from build123d import *

# Parameters (mm, degrees)
BOSS_EXTRUDE1_DEPTH = 100
SKETCH2_R           = 4
BOSS_EXTRUDE2_DEPTH = 5
CUT_EXTRUDE1_DEPTH  = 111.145358504
BOSS_EXTRUDE3_DEPTH = 20
SKETCH6_W           = 16
SKETCH6_H           = 82.013760225
CUT_EXTRUDE2_DEPTH  = 20
FILLET1_R           = 2
SKETCH7_W           = 20
SKETCH7_H           = 90.042878707
SKETCH7_W_2         = 16
SKETCH7_H_2         = 66.692206804
BOSS_EXTRUDE4_DEPTH = 15
CHAMFER1_SIZE       = 8


with BuildPart() as part:
    # Sketch1 → Boss-Extrude1 (new body)
    with BuildSketch(Plane.XY):
        Polygon((28, 4), (44, 4), (44, 9), (-16, 9), (-16, 4), (0, 4), (0, 0), (28, 0), align=None)
    extrude(amount=BOSS_EXTRUDE1_DEPTH)

    # Sketch2 → Boss-Extrude2 (add)
    with BuildSketch(Plane.XY.offset(100)):
        with BuildLine():
            Line((6, 15), (6, 0))
            Line((6, 0), (22, 0))
            Line((22, 0), (22, 15))
            ThreePointArc((22, 15), (14, 23), (6, 15))
        make_face()
        with Locations((14, 15)):
            Circle(SKETCH2_R, mode=Mode.SUBTRACT)
    extrude(amount=-BOSS_EXTRUDE2_DEPTH)

    # Sketch3 → Cut-Extrude1 (cut, through all)
    with BuildSketch(Plane(origin=(0, 9, 0), x_dir=(1, 0, 0), z_dir=(0, 1, 0))):
        Polygon((36, -100), (44, -88), (44, -100), align=None)
        Polygon((-8, -100), (-16, -100), (-16, -88), align=None)
    extrude(amount=-CUT_EXTRUDE1_DEPTH, mode=Mode.SUBTRACT)

    # Sketch5 → Boss-Extrude3 (add)
    with BuildSketch(Plane(origin=(0, 9, 0), x_dir=(1, 0, 0), z_dir=(0, 1, 0))):
        Polygon((-16, 0), (0, 0), (0, -5.756429966), (28.329099736, -5.756429966), (28.329099736, 0), (44, 0), (44, -12.986239775), (-16, -12.986239775), align=None)
    extrude(amount=BOSS_EXTRUDE3_DEPTH)

    # Sketch6 → Cut-Extrude2 (cut)
    with BuildSketch(Plane(origin=(0, 9, 0), x_dir=(1, 0, 0), z_dir=(0, 1, 0))):
        with Locations((14, -53.993119888)):
            Rectangle(SKETCH6_W, SKETCH6_H)
    extrude(amount=-CUT_EXTRUDE2_DEPTH, mode=Mode.SUBTRACT)

    # Fillet1
    fillet1_edges = [part.edges().sort_by_distance(p)[0] for p in [
        (6, 4.5, 12.986239775),
        (22, 4.5, 12.986239775),
        (22, 4.5, 95),
        (6, 4.5, 95),
    ]]
    fillet(fillet1_edges, radius=FILLET1_R)

    # Sketch7 → Boss-Extrude4 (add)
    with BuildSketch(Plane.XZ):
        with Locations((14, 52.847885125)):
            Rectangle(SKETCH7_W, SKETCH7_H)
        with Locations((14, 53.267861238)):
            Rectangle(SKETCH7_W_2, SKETCH7_H_2, mode=Mode.SUBTRACT)
    extrude(amount=BOSS_EXTRUDE4_DEPTH)

    # Chamfer1
    chamfer1_edges = [part.edges().sort_by_distance(p)[0] for p in [
        (4, -7.5, 97.869324478),
        (4, -7.5, 7.826445771),
        (24, -7.5, 7.826445771),
        (24, -7.5, 97.869324478),
    ]]
    chamfer(chamfer1_edges, length=CHAMFER1_SIZE)


solid = part.part
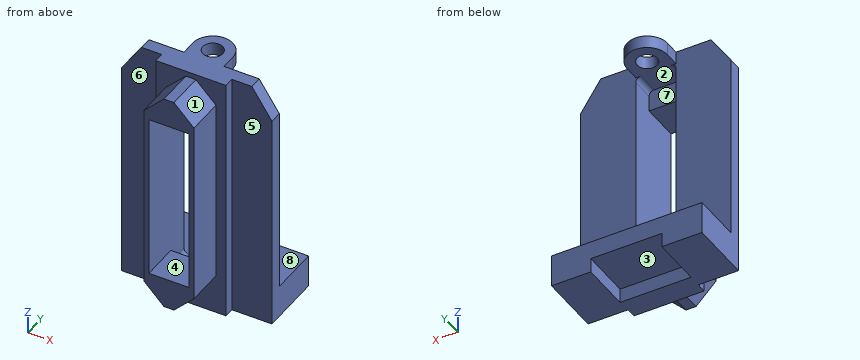
Check sheet for the modelled part. Datum: model origin and axes. Units: mm. Face numbers are marked on the shaded views. A direction names the side the tool comes from. Give positions to 0.01 mm unless a question says otherwise; leave off trailing zeros. Order: outer loops, then holes, each group sorted by start corner. A loop starts at its lowest first (then second) coordinate and runs counter-clockwise, first axis right, second up. Notation, with made-up numbers: (87.5, 71) - (116.5, 71) arc R22 cw to (116.5, 100) - close; hole circle Ø6 at (-28, 43.5). An arc over 180 degrees is marked (long way). Answer as CSV lines item,"result".
1. Section check B-B (x = 14). Record the boundary of the cut face in (y, z), then the cut area to 3 significant figures.
Result sheet:
outline,"(-15, 7.83) - (0, 7.83) - (0, 0) - (9, 0) - (9, 5.76) - (29, 5.76) - (29, 12.99) - (0, 12.99) - (0, 19.92) - (-15, 19.92) - close; (-15, 86.61) - (0, 86.61) - (0, 95) - (11, 95) - (11, 100) - (0, 100) - (0, 97.87) - (-15, 97.87) - close; (19, 95) - (23, 95) - (23, 100) - (19, 100) - close"
area,"687 mm²"
2. Section check A-A (y = -11.5). Record the boundary of the cut face in (x, z), then the cut area to 3 significant figures.
Result sheet:
outline,"(4, 15.83) - (12, 7.83) - (16, 7.83) - (24, 15.83) - (24, 89.87) - (16, 97.87) - (12, 97.87) - (4, 89.87) - close; hole (6, 19.92) - (22, 19.92) - (22, 86.61) - (6, 86.61) - close"
area,"606 mm²"
3. Section check D-D (y = 21). Record the boundary of the cut face in (x, z), then the cut area to 3 significant figures.
Result sheet:
outline,"(-16, 0) - (0, 0) - (0, 5.76) - (28.33, 5.76) - (28.33, 0) - (44, 0) - (44, 12.99) - (-16, 12.99) - close; (8.71, 95) - (19.29, 95) - (19.29, 100) - (8.71, 100) - close"
area,"669 mm²"
4. Go/stop test with flat-tipped pins: P1, Ø1, axis at x = 2.5, z = 30, coming from the -Y side; P2, Ø2, axis at x = 15, y = -6, coming from the +Z side; P3, Ø8, axis at y = -8, z = 82, coming from the +X side. Record where each tip stops, or that it passes through.
Result sheet:
P1,"y = 0"
P2,"z = 97.87"
P3,"x = 24"
5. Scan lines: probe 1 along Z at (x, y) = (13.5, 7.5); probe 2 along Y at (x, z) = (14, 97); probe 3 along Y at (x, z) = (14, 98). Record each from-to range of solid material in increasing order. Write a range as from..to.
Result sheet:
probe 1,"0..12.99, 95..100"
probe 2,"-15..11, 19..23"
probe 3,"0..11, 19..23"
6. Mould release check, pull along Y, two halves, no side actions. Record for the marked faces 6, 7 and 8: released by +Y, released by -Y, zero draft, split by the parting line, or undercut.
Result sheet:
face 6,"released by -Y"
face 7,"released by +Y"
face 8,"zero draft"
7. Tool access check on the marked faces 1, 2, 3, 4 and 5. Record the directions out of +Z, -Z, +X, -X, +Y, -Y that give a thin tool (end or side, any length) a straight path to the whole face; none if there is none.
Result sheet:
face 1,"+Z, +X, -Y"
face 2,"+Y"
face 3,"-Z, +Y"
face 4,"+Y, -Y"
face 5,"+Z, -Z, +X, -Y"
8. Section check C-C (z = 21). Record the boundary of the cut face in (x, y).
Result sheet:
outline,"(-16, 4) - (0, 4) - (0, 0) - (4, 0) - (4, -15) - (6, -15) - (6, 9) - (-16, 9) - close; (22, -15) - (24, -15) - (24, 0) - (28, 0) - (28, 4) - (44, 4) - (44, 9) - (22, 9) - close"
